Can you work these out from the model? Positions are in its coordinate system, mm. Face numbers are marked on the shaded views. A direction names the side the tool comes from. Coordinates: 2 decimals unless noted, no trailing zeros. Loops run counter-clockwise (first coordinate to the right, second up) from the corner with the lowest first, then second, coordinate; pieces in that order, holes last. Notation, with made-up numbers: M 5.5,-16.75 L 21.5,-16.75 A25 cw 21.5,13.25 Z; hole C -31.5,-23.5 d8. An arc over 180 degrees is marked long. Return JSON: item names as keys, results as strings. Group by question number.
```python
from build123d import *

# Parameters (mm, degrees)
CROQUIS1_W              = 196
CROQUIS1_H              = 78
SALIENTE_EXTRUIR1_DEPTH = 5
CROQUIS2_W              = 10
CROQUIS2_H              = 7
SALIENTE_EXTRUIR2_DEPTH = 200
SALIENTE_EXTRUIR3_DEPTH = 200
SALIENTE_EXTRUIR4_DEPTH = 2
CORTAR_EXTRUIR2_DEPTH   = 10


with BuildPart() as part:
    # Croquis1 → Saliente-Extruir1 (new body)
    with BuildSketch(Plane(origin=(0, 0, 0), x_dir=(1, 0, 0), z_dir=(0, 1, 0))):
        with Locations((-48.059642147, -1)):
            Rectangle(CROQUIS1_W, CROQUIS1_H)
    extrude(amount=SALIENTE_EXTRUIR1_DEPTH)

    # Croquis2 → Saliente-Extruir2 (add)
    with BuildSketch(Plane(origin=(0, 5, 0), x_dir=(1, 0, 0), z_dir=(0, 1, 0))):
        with Locations((-139.059642147, -34.5)):
            Rectangle(CROQUIS2_W, CROQUIS2_H)
        with Locations((42.940357853, -34.5)):
            Rectangle(CROQUIS2_W, CROQUIS2_H)
    extrude(amount=SALIENTE_EXTRUIR2_DEPTH)

    # Croquis4 → Saliente-Extruir3 (add)
    with BuildSketch(Plane(origin=(0, 5, 0), x_dir=(1, 0, 0), z_dir=(0, 1, 0))):
        Polygon((-146.059642147, -23), (-134.059642147, -23), (-134.059642147, -40), (37.940357853, -40), (37.940357853, -24.127895053), (49.940357853, -24.127895053), (49.940357853, 38), (47.940357853, 38), (47.940357853, -22.127895053), (35.940357853, -22.127895053), (35.940357853, -38), (-132.059642147, -38), (-132.059642147, -21.170903905), (-144.059642147, -21.170903905), (-144.059642147, 38), (-146.059642147, 38), align=None)
    extrude(amount=SALIENTE_EXTRUIR3_DEPTH)

    # Croquis5 → Saliente-Extruir4 (add)
    with BuildSketch(Plane(origin=(0, 205, 0), x_dir=(1, 0, 0), z_dir=(0, 1, 0))):
        Polygon((-146.059642147, 38), (49.940357853, 38), (49.940357853, -24.127895053), (37.940357853, -24.127895053), (37.940357853, -40), (-134.059642147, -40), (-134.059642147, -23), (-146.059642147, -23), align=None)
    extrude(amount=SALIENTE_EXTRUIR4_DEPTH)

    # Croquis6 → Cortar-Extruir2 (cut)
    with BuildSketch(Plane.XZ):
        with BuildLine():
            Line((-83.059642147, 9), (-13.059642147, 9))
            ThreePointArc((-13.059642147, 9), (-5.059642147, 1), (-13.059642147, -7))
            Line((-13.059642147, -7), (-83.059642147, -7))
            ThreePointArc((-83.059642147, -7), (-91.059642147, 1), (-83.059642147, 9))
        make_face()
    extrude(amount=-CORTAR_EXTRUIR2_DEPTH, mode=Mode.SUBTRACT)


solid = part.part
```
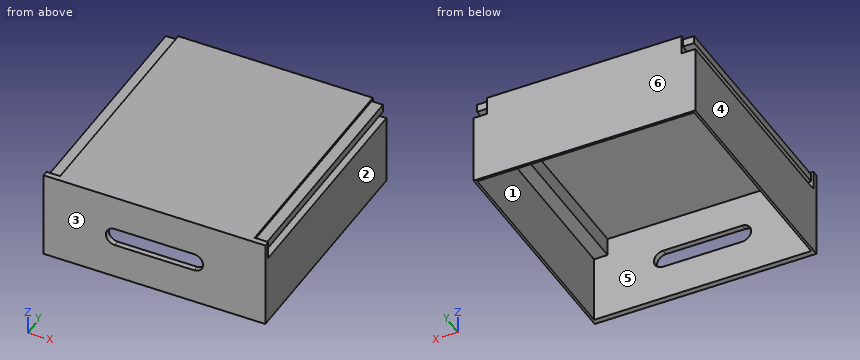
1) Suppose I cut it at B-B, the plane z = -24. List the corners of the cut face in (x, y) for me, then the cut area to 3 significant figures.
2) For the marked faces 1 and 2, which set-ups out of +Z, -Z, +X, -X, +Y, -Y let a thin tool reach every point of the face, with its end or its side?
3) If we mould it in two halves opening along Y, with no side actions, what happens to the marked faces 3, 4, 5 and 6? For each: +Y half, -Y half, draft (parallel to the pull), parting line (faces both ways), or undercut.
4) For pin 1 (3.5 mm diameter, centred on x = 43.5, z = 36, fed in from +Y); pin 2 (8 mm diameter, centred on y = 161.5, z = 30, fed in from -X); pin 3 (5 mm diameter, centred on x = -141, y = 116.5, fed in from -Z), each with a flat end and sliding along its axis, tell me the tip position at first contact or that it passes through.
5) If I drill on line 1 (Y direction, x = -91, z = -31.5); line 2 (X direction, y = 193.5, z = -14); line 3 (Z direction, x = 34.5, y = 190.5), over which ranges is the centre line in solid material (lowest first)? Write a range as from..to.
6) Suppose I cut it at A-A, the plane x = -22.5. List the corners of the cut face in (y, z) for me, then the cut area to 3 significant figures.
7) Suppose I cut it at C-C, the plane z = 1. List the corners of the cut face in (x, y) for me, then the cut area to 3 significant figures.
8) Suppose I cut it at D-D, the plane y = 60. List the corners of the cut face in (x, z) for me, then the cut area to 3 significant figures.
Returned:
{
 "1": {"outline": "M -146.06,0 L 49.94,0 L 49.94,207 L -146.06,207 Z; hole M -144.06,5 L 47.94,5 L 47.94,205 L -144.06,205 Z", "area": "2,170 mm²"},
 "2": {"face 1": "-Z", "face 2": "+Z, -Z, +X, +Y, -Y"},
 "3": {"face 3": "-Y half", "face 4": "draft", "face 5": "undercut", "face 6": "+Y half"},
 "4": {"pin 1": "stops at y = 205", "pin 2": "stops at x = -144.06", "pin 3": "stops at z = 21.17"},
 "5": {"line 1": "y = 0..5, 205..207", "line 2": "x = -146.06..-144.06, 47.94..49.94", "line 3": "z = 38..40"},
 "6": {"outline": "M 0,-38 L 5,-38 L 5,-7 L 0,-7 Z; M 0,9 L 5,9 L 5,38 L 205,38 L 205,-38 L 207,-38 L 207,40 L 0,40 Z", "area": "866 mm²"},
 "7": {"outline": "M -146.06,0 L -91.06,0 L -91.06,5 L -144.06,5 L -144.06,205 L 47.94,205 L 47.94,5 L -5.06,5 L -5.06,0 L 49.94,0 L 49.94,207 L -146.06,207 Z", "area": "1,740 mm²"},
 "8": {"outline": "M -146.06,-38 L -144.06,-38 L -144.06,21.17 L -132.06,21.17 L -132.06,38 L 35.94,38 L 35.94,22.13 L 47.94,22.13 L 47.94,-38 L 49.94,-38 L 49.94,24.13 L 37.94,24.13 L 37.94,31 L 47.94,31 L 47.94,38 L 37.94,38 L 37.94,40 L -134.06,40 L -134.06,38 L -144.06,38 L -144.06,31 L -134.06,31 L -134.06,23 L -146.06,23 Z", "area": "834 mm²"}
}
